Geometry: final body of the model. Coordinates: model frame, mm. Face numbers are marked on the shaded views. Coordinates: 2 decimals unless noted, no trailing zeros. Loops run counter-clockwise (first coordinate to the right, second up) from the corner with the lowest first, then second, coordinate; pieces in that order, holes last. Notation, with made-up numbers: (56, -31.75) - (115, -31.75) arc R13 ccw to (115, -10.75) - close; hole circle Ø8 at (29, -9.75). An arc over 180 degrees is marked (long way). Return JSON: item names as keys, results as strings.
Autodesk Inventor part; units mm, degrees
ref_plane "YZ Plane" through (0, 0, 0) normal (1, 0, 0) x (0, 1, 0)
ref_plane "XZ Plane" through (0, 0, 0) normal (0, 1, 0) x (-1, 0, 0)
ref_plane "XY Plane" through (0, 0, 0) normal (0, 0, 1) x (1, 0, 0)
sketch "Sketch1" plane through (0, 0, 0) normal (0, 1, 0) x (-1, 0, 0)
  line L0 (-50, -50) -> (50, -50) construction
  line L1 (50, -50) -> (50, 50) construction
  line L2 (50, 50) -> (-50, 50) construction
  line L3 (-50, 50) -> (-50, -50) construction
  line L4 (-50, -50) -> (50, 50) construction
  line L5 (50, -50) -> (-50, 50) construction
  circle A0 centre (0, 0) radius 50
  dimension "d0" = 100
  dimension "d8" = 100
extrude "Extrusion1" add sketch "Sketch1" along normal blind 2
sketch "Sketch2" plane through (0, 2, 0) normal (0, 1, 0) x (1, 0, 0)
  circle A0 centre (0, 0) radius 50
  circle A1 centre (0, 0) radius 47
  dimension "d9" = 3
extrude "Extrusion2" add sketch "Sketch2" along normal blind 17
fillet "Fillet1" radius 2 2 edges at (-47, 2, 0) (50, 0, 0)
properties part number "Petri"
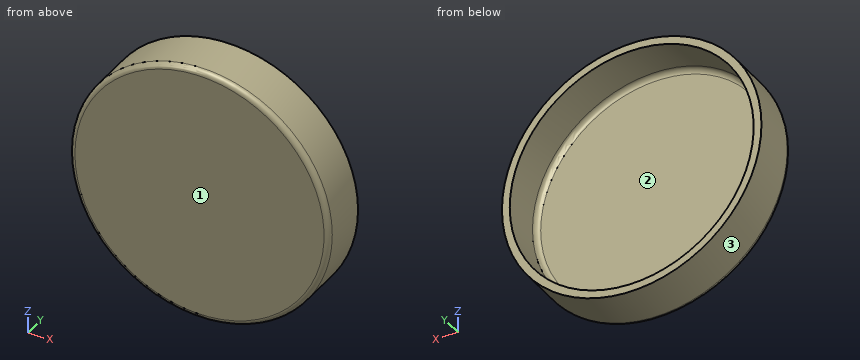
Item 1: First-contact query: pin 1 Ø2 at (x, z) = (10.5, 25.5) entering from +Y; pin 2 Ø10 at (x, y) = (26.5, 17) entering from +Z; pin 3 Ø3 at (x, y) = (22, 4) entering from +Z. Flat tips, straight axial feed; report the tip coordinate or a pass-through.
Worked out:
{"pin 1": "y = 2", "pin 2": "z = 45.14", "pin 3": "z = 45.6"}
Item 2: Ray query, probe 1 along Z at (x, y) = (0, 13.5); probe 2 along Y at (x, z) = (17, -17.5). Return the intervals inside material, ascending. Write a range as from..to.
Worked out:
{"probe 1": "-50..-47, 47..50", "probe 2": "0..2"}
Item 3: Mould query, pull axis X, two halves, no side actions, for the marked faces 1, 2 and 3. Classes: +X half, -X half, draft (parallel to the pull), parting line (faces both ways), or undercut.
Worked out:
{"face 1": "draft", "face 2": "undercut", "face 3": "parting line"}
Item 4: Section query A-A, the plane y = 6.75. Return loops of the section in (x, z).
Worked out:
{"outline": "circle Ø100 at (0, 0); hole circle Ø94 at (0, 0)"}
